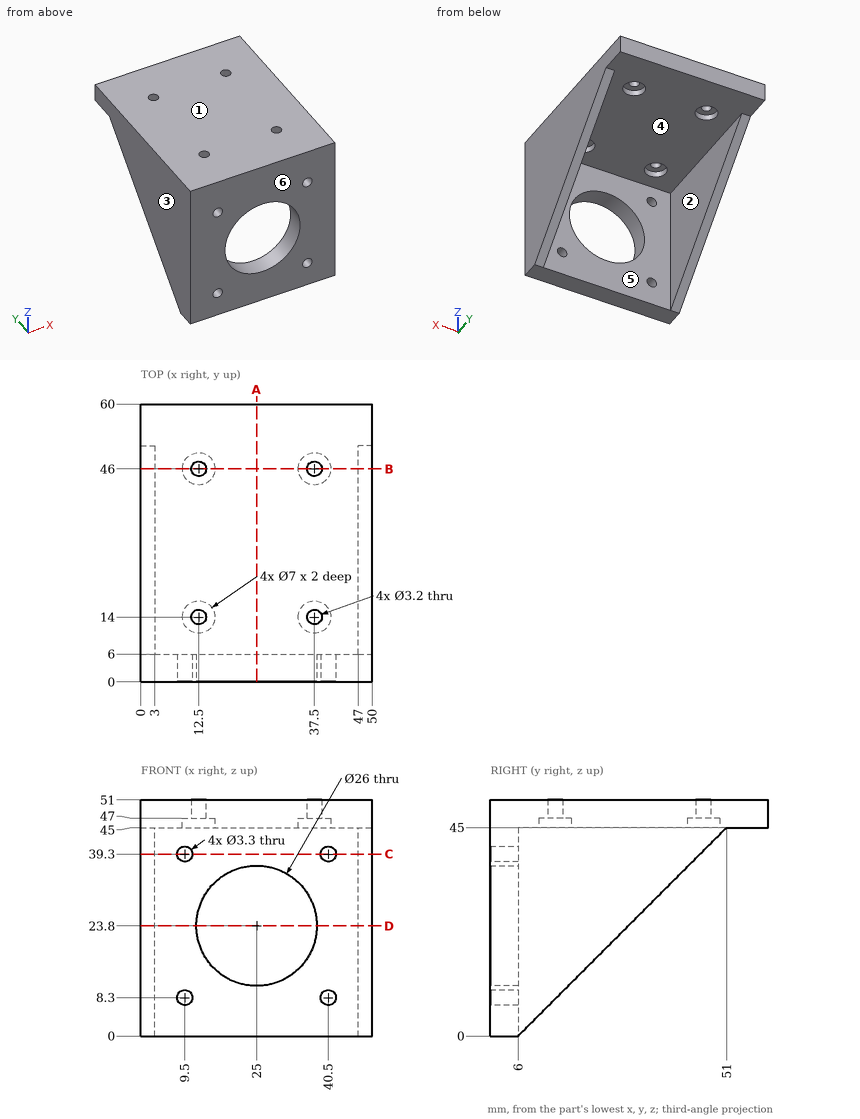
The drawing under review shows one solid part. Ordinate dimensions are in mm from its lowest x, y, z. A direction names the side the tool comes from. Coordinates: 2 decimals unless noted, no trailing zeros. Write each loop counter-clockwise with the first axis right and the second up, starting at its lowest first coordinate (ties: lowest second). Pieces come first, ordered by that corner, then holes. Notation, with made-up numbers: (70, -34) - (84, -34) arc R25 ccw to (84, 0) - close; hole circle Ø3 at (5, -10). An arc over 180 degrees is marked (long way). Put each result on its own line as item: value.
1. Mouldability with a two-part tool opening along X and no side actions: class the marked faces 1, 2, 3 and 4 as released by +X, released by -X, zero draft, split by the parting line, or undercut.
Values found:
face 1: zero draft
face 2: undercut
face 3: released by -X
face 4: undercut
2. Add section B-B, the plane y = 46. Give the boundary of the cut face in (x, z).
Values found:
outline: (0, 40) - (3, 40) - (3, 45) - (9, 45) - (9, 47) - (10.9, 47) - (10.9, 51) - (0, 51) - close; (14.1, 47) - (16, 47) - (16, 45) - (34, 45) - (34, 47) - (35.9, 47) - (35.9, 51) - (14.1, 51) - close; (39.1, 47) - (41, 47) - (41, 45) - (47, 45) - (47, 40) - (50, 40) - (50, 51) - (39.1, 51) - close
3. Add section A-A, the plane x = 25. Give the boundary of the cut face in (y, z), then the cut area to 3 significant figures.
Values found:
outline: (0, 0) - (6, 0) - (6, 10.8) - (0, 10.8) - close; (0, 36.8) - (6, 36.8) - (6, 45) - (60, 45) - (60, 51) - (0, 51) - close
area: 474 mm²
4. Add section C-C, the plane z = 39.3. Give the boundary of the cut face in (x, y), then the cut area to 3 significant figures.
Values found:
outline: (0, 0) - (7.85, 0) - (7.85, 6) - (3, 6) - (3, 45.3) - (0, 45.3) - close; (11.15, 0) - (38.85, 0) - (38.85, 6) - (11.15, 6) - close; (42.15, 0) - (50, 0) - (50, 45.3) - (47, 45.3) - (47, 6) - (42.15, 6) - close
area: 496 mm²
5. Machinability: for the marked faces 5 and 6, which of the approach directions +Z, -Z, +X, -X, +Y, -Y give a long, thin tool a straight path to every point of the face, cutting with its end or side? Answer none if there is none.
Values found:
face 5: -Z, +Y
face 6: +Z, -Z, +X, -X, -Y
6. Add section D-D, the plane z = 23.8. Give the boundary of the cut face in (x, y).
Values found:
outline: (0, 0) - (12, 0) - (12, 6) - (3, 6) - (3, 29.8) - (0, 29.8) - close; (38, 0) - (50, 0) - (50, 29.8) - (47, 29.8) - (47, 6) - (38, 6) - close
7. Wall thickness on probe 1 along X at (y, z) = (2.5, 8.3); probe 2 along X at (y, z) = (42.5, 38.5); probe 3 along Z at (x, y) = (9, 2): over which ranges is each line inside the solid? List them lowest first.
Values found:
probe 1: 0 to 7.85, 11.15 to 38.85, 42.15 to 50
probe 2: 0 to 3, 47 to 50
probe 3: 0 to 6.73, 9.87 to 37.73, 40.87 to 51
8. For pin 1 (4 mm diameter, centred on x = 37.5, y = 14, fed in from -Z); pin 2 (9 mm diameter, centred on x = 37.5, y = 46, fed in from -Z); pin 3 (4 mm diameter, centred on x = 24.5, z = 38.5, fed in from +Y), all flat-tipped, find the tip position at first contact; note any pin that passes through.
Values found:
pin 1: z = 47
pin 2: z = 45
pin 3: y = 6
